Source: CAD feature listing. Evaluate the final solid. Frame: model axes, mm. Face numbers are marked on the shaded views. Give positions to 0.01 mm unless a question says otherwise; leave off trailing zeros. Loops run counter-clockwise (first coordinate to the right, second up) from the corner with the lowest first, then second, coordinate; pieces in that order, holes last.
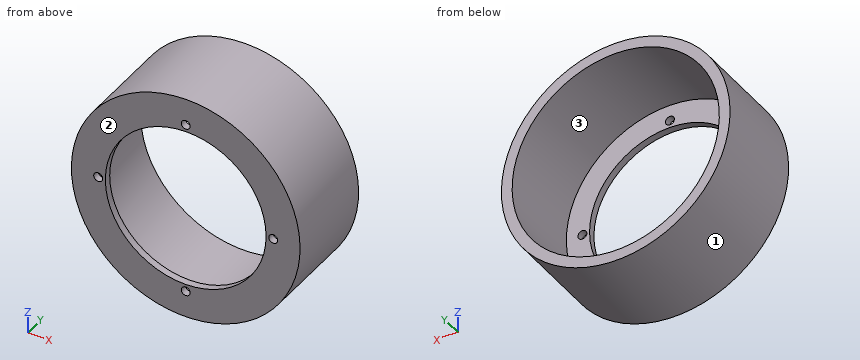
from build123d import *

# Parameters (mm, degrees)
SKETCH_1_R               = 32
EXTRUDE_1_DEPTH          = 27
CUT_EXTRUDE_3_DEPTH      = 51.318982502
CUT_EXTRUDE_3_DEPTH_BACK = 51.318982502
SKETCH_5_R               = 22.5
SKETCH_6_R               = 29
CUT_EXTRUDE_4_DEPTH      = 25
HOLE_WIZARD_M3_1_D       = 2.5


with BuildPart() as part:
    # 草图1 → 凸台-拉伸1 (new body)
    with BuildSketch(Plane(origin=(0, 0, 0), x_dir=(1, 0, 0), z_dir=(0, 1, 0))):
        with Locations(Location((0, 0, 0), (0, 0, 270))):
            Circle(SKETCH_1_R)
    extrude(amount=EXTRUDE_1_DEPTH)

    # 草图5 → 切除-拉伸3 (cut, two sides: drawn at the far end of the back side and taken through both)
    with BuildSketch(Plane(origin=(0, 5, 0), x_dir=(-1, 0, 0), z_dir=(0, -1, 0)).offset(-CUT_EXTRUDE_3_DEPTH_BACK)):
        with Locations(Location((0, 0, 0), (0, 0, 90))):
            Circle(SKETCH_5_R)
    extrude(amount=CUT_EXTRUDE_3_DEPTH + CUT_EXTRUDE_3_DEPTH_BACK, mode=Mode.SUBTRACT)

    # 草图6 → 切除-拉伸4 (cut)
    with BuildSketch(Plane(origin=(0, 27, 0), x_dir=(1, 0, 0), z_dir=(0, 1, 0))):
        with Locations(Location((0, 0, 0), (0, 0, 270))):
            Circle(SKETCH_6_R)
    extrude(amount=-CUT_EXTRUDE_4_DEPTH, mode=Mode.SUBTRACT)

    # M3 螺纹孔1 (through all)
    with Locations(Plane(origin=(0, 0, 0), x_dir=(-1, 0, 0), z_dir=(0, -1, 0))):
        with Locations((24.5, 0), (0, 24.5), (-24.5, 0), (0, -24.5)):
            Hole(HOLE_WIZARD_M3_1_D / 2)


solid = part.part
1) Pull-direction query (Z, two-part tool) for the marked faces 1, 2 and 3; classes: released by +Z, released by -Z, zero draft, split by the parting line, or undercut.
Checks:
face 1: split by the parting line
face 2: zero draft
face 3: undercut
2) Contact query for flat-ended pins moving along their axis: P1, Ø8, axis at x = -16.5, z = -9, coming from the +Y side; P2, Ø1, axis at x = 20, y = 6.5, coming from the +Z side; P3, Ø2, axis at y = 13, z = -20.5, coming from the -X side. Output: stop coordinate, or through.
Checks:
P1: stops at y = 2
P2: stops at z = 25.37
P3: stops at x = -25.37
3) Ray query, probe 1 along Z at (x, y) = (-21, 23.5); probe 2 along Z at (x, y) = (-2.5, 25); probe 3 along X at (y, z) = (8.75, 6). Return the intervals inside material, ascending.
Checks:
probe 1: z = -24.15 to -20, 20 to 24.15
probe 2: z = -31.9 to -28.89, 28.89 to 31.9
probe 3: x = -31.43 to -28.37, 28.37 to 31.43
4) Cut plane A-A (x = 17). Return loops of the section in (y, z), and give its area (3 significant figures).
Checks:
outline: (0, -27.11) - (27, -27.11) - (27, -23.49) - (2, -23.49) - (2, -14.74) - (0, -14.74) - close; (0, 14.74) - (2, 14.74) - (2, 23.49) - (27, 23.49) - (27, 27.11) - (0, 27.11) - close
area: 230 mm2
5) Cut plane C-C (y = 22.25). Return loops of the section in (x, z), and give its area (3 significant figures).
Checks:
outline: circle Ø64 at (0, 0); hole circle Ø58 at (0, 0)
area: 575 mm2
6) Cut plane B-B (z = 16). Return loops of the section in (x, y), and give its area (3 significant figures).
Checks:
outline: (-27.71, 0) - (-15.82, 0) - (-15.82, 2) - (-24.19, 2) - (-24.19, 27) - (-27.71, 27) - close; (15.82, 0) - (27.71, 0) - (27.71, 27) - (24.19, 27) - (24.19, 2) - (15.82, 2) - close
area: 224 mm2
